Design review of the part built by this model. Coordinates are the model's own, in mm. A direction names the side the tool comes from. Give positions to 0.01 mm unless a question says otherwise; leave off trailing zeros. Loops run counter-clockwise (first coordinate to the right, second up) from the corner with the lowest first, then second, coordinate; pieces in that order, holes last. Notation, with made-up numbers: M 22,41 L 64,41 A19 cw 64,47 Z; hole C -13,-25.5 d6. An arc over 180 degrees is marked long. Use a Markdown table: item, result. Add a question column.
(1) For faces 1 (the face through (-1, 5, -150)), 2 (the face through (101, 6, 126)), list the 3-axis set-ups (+Z, -Z, +X, -X, +Y, -Y) from which the entire face can be reached by the end or side of a thin tool; tool diameter is ignored.
(2) Draft analysis for pull direction X (two halves, no side actions). For faces 3 (the face through (-156.11, 5.07, 127.45)), 4 (the face through (52.857, 4.93, 121.748)), 5 (the face through (-1, 5, 150)), state which applies: pulls with the +X half, pulls with the -X half, needs draft (parallel to the pull), parting line crosses it, or undercut.
(3) Add section A-A, the plane x = 67.5. Give the boundary of the cut face in (y, z), then the cut area to 3 significant figures.
(4) Insertion check: pin 1 Ø6 at (x, z) = (99.2, 123.9) entering from +Y. The pin has a flat end and moves straight along its axis. Give the tip position at first contact, or say it passes through.
(5) Add section B-B, the plane y = 3.25. State how many separate pieces and enclosed holes the cut face has, then the cut area to 3 significant figures.
(6) For probe 1 along X at (y, z) = (7.75, -100); probe 2 along X at (y, z) = (5.25, -125.5); probe 3 along Z at (x, y) = (112.2, 8.7), list the stretches that pass through material, from the lowest coordinate up.
```python
from build123d import *

# Parameters (mm, degrees)
SKETCH11_W                     = 355
SKETCH11_H                     = 300
SKETCH11_R                     = 15
BOSS_EXTRUDE2_DEPTH            = 10
CBORE_FOR_M4_SHCS2_D           = 4.5
CBORE_FOR_M4_SHCS2_CBORE_D     = 8
CBORE_FOR_M4_SHCS2_CBORE_DEPTH = 4
F_3_2_3_2_DIAMETER_HOLE2_D     = 3.2
M4_CLEARANCE_HOLE1_OUTLINE_R   = 2.25
M4_CLEARANCE_HOLE1_DEPTH       = 10
M4_CLEARANCE_HOLE2_D           = 4.5
FILLET1_R                      = 75


# Read off the part's stored shape, not the designer's step: M4 Clearance Hole1
with BuildPart() as part:
    # Sketch11 → Boss-Extrude2 (new body)
    with BuildSketch(Plane(origin=(0, 0, 0), x_dir=(1, 0, 0), z_dir=(0, 1, 0))):
        Rectangle(SKETCH11_W, SKETCH11_H)
        with Locations(Location((67.5, -125, 0), (0, 0, 270))):
            Circle(SKETCH11_R, mode=Mode.SUBTRACT)
        with Locations(Location((67.5, 125, 0), (0, 0, 270))):
            Circle(SKETCH11_R, mode=Mode.SUBTRACT)
    extrude(amount=BOSS_EXTRUDE2_DEPTH)

    # CBORE for M4 SHCS2 (through all)
    with Locations(Plane(origin=(0, 10, 0), x_dir=(1, 0, 0), z_dir=(0, 1, 0))):
        with Locations((99.2, 123.9), (112.2, 123.9), (112.2, -123.9), (99.2, -123.9)):
            CounterBoreHole(CBORE_FOR_M4_SHCS2_D / 2, CBORE_FOR_M4_SHCS2_CBORE_D / 2, CBORE_FOR_M4_SHCS2_CBORE_DEPTH)

    # Ø3.2 (3.2) Diameter Hole2 (through all)
    with Locations(Plane(origin=(0, 10, 0), x_dir=(1, 0, 0), z_dir=(0, 1, 0))):
        with Locations((132.110460528, 46.535002739), (112.111563058, 46.745002739), (110.841563058, -1.514997261), (132.110460528, -1.514997261), (60.041563058, 13.725002739), (60.041563058, 41.665002739)):
            Hole(F_3_2_3_2_DIAMETER_HOLE2_D / 2)

    # M4 Clearance Hole1 outline → M4 Clearance Hole1 (cut)
    with BuildSketch(Plane(origin=(0, 0, 0), x_dir=(1, 0, 0), z_dir=(0, 1, 0))):
        with Locations((137.5, 100)):
            Circle(M4_CLEARANCE_HOLE1_OUTLINE_R)
        with Locations((-137.5, -100)):
            Circle(M4_CLEARANCE_HOLE1_OUTLINE_R)
        with Locations((-137.5, 100)):
            Circle(M4_CLEARANCE_HOLE1_OUTLINE_R)
        with Locations((137.5, -100)):
            Circle(M4_CLEARANCE_HOLE1_OUTLINE_R)
        Circle(M4_CLEARANCE_HOLE1_OUTLINE_R)
    extrude(amount=M4_CLEARANCE_HOLE1_DEPTH, mode=Mode.SUBTRACT)

    # M4 Clearance Hole2 (through all)
    with Locations(Plane(origin=(0, 10, 0), x_dir=(1, 0, 0), z_dir=(0, 1, 0))):
        with Locations((-80.554499739, -118.9), (-80.554499739, 118.9)):
            Hole(M4_CLEARANCE_HOLE2_D / 2)

    # Fillet1
    fillet1_edges = [part.edges().sort_by_distance(p)[0] for p in [
        (177.5, 5, -150),
        (177.5, 5, 150),
        (-177.5, 5, 150),
        (-177.5, 5, -150),
    ]]
    fillet(fillet1_edges, radius=FILLET1_R)


solid = part.part
```
Established:
| question | item | result |
|---|---|---|
| 1 | face 1 | -Z, +X, -X, +Y, -Y |
| 1 | face 2 | +Y |
| 2 | face 3 | pulls with the -X half |
| 2 | face 4 | undercut |
| 2 | face 5 | needs draft |
| 3 | outline | M 0,-150 L 10,-150 L 10,-140 L 0,-140 Z; M 0,-110 L 10,-110 L 10,110 L 0,110 Z; M 0,140 L 10,140 L 10,150 L 0,150 Z |
| 3 | area | 2,400 mm^2 |
| 4 | pin 1 | y = 6 |
| 5 | separate pieces | 1 |
| 5 | enclosed holes | 19 |
| 5 | area | 100,000 mm^2 |
| 6 | probe 1 | -173.21 to -139.75, -135.25 to 135.25, 139.75 to 173.21 |
| 6 | probe 2 | -157.95 to 52.51, 82.49 to 97.62, 100.78 to 110.62, 113.78 to 157.95 |
| 6 | probe 3 | -149.37 to -127.9, -119.9 to -48.34, -45.15 to 0.67, 2.36 to 119.9, 127.9 to 149.37 |
